from build123d import *
from OCP.BRepAlgoAPI import BRepAlgoAPI_Cut
from OCP.TopTools import TopTools_ListOfShape

# Parameters (mm, degrees)
SKETCH1_R               = 10
BOSS_EXTRUDE2_DEPTH     = 30
SKETCH4_R               = 10
CUT_EXTRUDE1_DEPTH      = 15
CHAMFER1_SIZE           = 20
CUT_EXTRUDE2_DEPTH      = 174.638139858
CUT_EXTRUDE2_DEPTH_BACK = 174.638139858
BOSS_EXTRUDE3_DEPTH     = 45
CUT_EXTRUDE3_DEPTH      = 198.547978004
CUT_EXTRUDE3_DEPTH_BACK = 15
SKETCH6_3_R             = 9
SKETCH8_W               = 15
SKETCH8_H               = 36
BOSS_EXTRUDE4_DEPTH     = 45.000002
SKETCH10_R              = 9
CUT_EXTRUDE4_DEPTH      = 198.547978004
BOSS_EXTRUDE5_DEPTH     = 10
CHAMFER2_SIZE           = 12
CUT_EXTRUDE5_DEPTH      = 40
CUT_EXTRUDE6_DEPTH      = 217.852953896
CUT_EXTRUDE6_DEPTH_BACK = 217.852953896
SKETCH14_W              = 100
SKETCH14_H              = 60
CUT_EXTRUDE7_DEPTH      = 145.655593904
CUT_EXTRUDE7_DEPTH_BACK = 10
SKETCH16_R              = 10
CUT_EXTRUDE8_DEPTH      = 15


# Some blends are built 0.0001 mm under size
with BuildPart() as part:
    # Sketch1 → Boss-Extrude2 (new, symmetric)
    # profile 1 of 3: a face of its own
    with BuildSketch(Plane.XY):
        Polygon((25, -10), (-4.997737685, -45.002262315), (-25, -25), (-25, 25), (25, 25), align=None)
        Circle(SKETCH1_R, mode=Mode.SUBTRACT)
    # profile 2 of 3: a face of its own
    with BuildSketch(Plane.XY):
        Polygon((45, -10), (25, -10), (-4.997737685, -45.002262315), (45.002262315, -45.002262315), (75, -41.079226753), (75, -2.548159698), align=None)
    # profile 3 of 3: a face of its own
    with BuildSketch(Plane.XY):
        Polygon((130, 11.113547523), (75, -2.548159698), (75, -41.079226753), (130, -33.886452477), (165, -33.886452477), (165, 11.113547523), align=None)
    extrude(amount=BOSS_EXTRUDE2_DEPTH, both=True)

    # Sketch4 → Cut-Extrude1 (cut, symmetric)
    with BuildSketch(Plane.XY):
        Polygon((25, -10), (-4.997737685, -45.002262315), (-25, -25), (-25, 25), (25, 25), align=None)
        Circle(SKETCH4_R, mode=Mode.SUBTRACT)
    extrude(amount=CUT_EXTRUDE1_DEPTH, both=True, mode=Mode.SUBTRACT)

    # Chamfer1
    chamfer1_edges = [part.edges().sort_by_distance(p)[0] for p in [
        (25, -10, -22.5),
        (25, -10, 22.5),
    ]]
    chamfer(chamfer1_edges, length=CHAMFER1_SIZE - 0.0001)  # a hair under: the kernel refuses the full size

    # Sketch5 → Cut-Extrude2 (cut, two sides: drawn at the far end of the back side and taken through both)
    with BuildSketch(Plane(origin=(0, 0, 0), x_dir=(1, 0, 0), z_dir=(0, 1, 0)).offset(-CUT_EXTRUDE2_DEPTH_BACK)):
        Polygon((165, -30), (165, -18), (55.074227224, -30), align=None)
        Polygon((165, 18), (165, 30), (55.074227224, 30), align=None)
    extrude(amount=CUT_EXTRUDE2_DEPTH + CUT_EXTRUDE2_DEPTH_BACK, mode=Mode.SUBTRACT)

    # Sketch6 → Boss-Extrude3 (add)
    with BuildSketch(Plane(origin=(165, 0, 0), x_dir=(0, 0, -1), z_dir=(1, 0, 0))):
        with BuildLine():
            Line((-18, -33.886452477), (18, -33.886452477))
            Line((18, -33.886452477), (18, -17.886452477))
            ThreePointArc((18, -17.886452477), (0, -25.375680921), (-18, -17.886452477))
            Line((-18, -17.886452477), (-18, -33.886452477))
        make_face()
    extrude(amount=BOSS_EXTRUDE3_DEPTH)

    # Sketch6<3> → Cut-Extrude3 (cut, two sides: drawn at the far end of the back side and taken through both)
    with BuildSketch(Plane(origin=(165, 0, 0), x_dir=(0, 0, -1), z_dir=(1, 0, 0)).offset(-CUT_EXTRUDE3_DEPTH_BACK)):
        with Locations(Location((0, -1.886452477, 0), (0, 0, 90))):
            Circle(SKETCH6_3_R)
    extrude(amount=CUT_EXTRUDE3_DEPTH + CUT_EXTRUDE3_DEPTH_BACK, mode=Mode.SUBTRACT)

    # Sketch8 → Boss-Extrude4 (add)
    with BuildSketch(Plane.XZ.offset(33.886452477)):
        with Locations((202.5, 0)):
            Rectangle(SKETCH8_W, SKETCH8_H)
    extrude(amount=-BOSS_EXTRUDE4_DEPTH)

    # Sketch10 → Cut-Extrude4 (cut, through all)
    with BuildSketch(Plane(origin=(165, 0, 0), x_dir=(0, 0, -1), z_dir=(1, 0, 0))):
        with Locations(Location((0, -1.886452477, 0), (0, 0, 90))):
            Circle(SKETCH10_R)
    extrude(amount=CUT_EXTRUDE4_DEPTH, mode=Mode.SUBTRACT)

    # Sketch11 → Boss-Extrude5 (add)
    with BuildSketch(Plane.XZ.offset(33.886452477)):
        Polygon((130, 21.82076004), (130, -21.82076004), (165, -18), (210, -18), (210, 18), (165, 18), align=None)
    extrude(amount=BOSS_EXTRUDE5_DEPTH)

    # Chamfer2
    # the kernel refuses this chamfer: 12 mm, written as the material it takes off along each edge
    with BuildSketch(Plane(origin=(130, -43.886452477, 52.680955896), x_dir=(0, 1, 0), z_dir=(0, 0, -1))) as chamfer2_piece_1_section:
        Polygon((CHAMFER2_SIZE, 0), (0, CHAMFER2_SIZE), (0, 0), align=None)
    chamfer2_piece_1 = extrude(amount=105.361911791, mode=Mode.PRIVATE)
    chamfer2_piece_1 = split(chamfer2_piece_1, bisect_by=Plane(origin=(128.714213423, -34.054604706, 52.680955896), z_dir=(0.1296735244167249, -0.9915567442488328, 0)), keep=Keep.TOP, mode=Mode.PRIVATE)
    add(chamfer2_piece_1, mode=Mode.SUBTRACT)

    # Sketch13 → Cut-Extrude5 (cut)
    with BuildSketch(Plane.XY.offset(18)):
        with BuildLine():
            Line((165, -17.886452477), (195, -17.886452477))
            ThreePointArc((195, -17.886452477), (180, -25.224548687), (165, -17.886452477))
        make_face()
    extrude(amount=-CUT_EXTRUDE5_DEPTH, mode=Mode.SUBTRACT)

    # Sketch14 → Cut-Extrude6 (cut, two sides: drawn at the far end of the back side and taken through both)
    with BuildSketch(Plane(origin=(0, 0, 0), x_dir=(1, 0, 0), z_dir=(0, 1, 0)).offset(-CUT_EXTRUDE6_DEPTH_BACK)):
        with Locations((25, 0)):
            Rectangle(SKETCH14_W, SKETCH14_H)
    extrude(amount=CUT_EXTRUDE6_DEPTH + CUT_EXTRUDE6_DEPTH_BACK, mode=Mode.SUBTRACT)

    # Sketch16 → Cut-Extrude7 (cut, two sides: drawn at the far end of the back side and taken through both)
    with BuildSketch(Plane.ZY.offset(-75).offset(-CUT_EXTRUDE7_DEPTH_BACK)):
        with Locations(Location((0, -20.03233432, 0), (0, 0, 180))):
            Circle(SKETCH16_R)
    extrude(amount=CUT_EXTRUDE7_DEPTH + CUT_EXTRUDE7_DEPTH_BACK, mode=Mode.SUBTRACT)


with BuildPart() as cut_extrude8_tool:
    # Sketch17 → Cut-Extrude8 (new body)
    with BuildSketch(Plane(origin=(210, 0, 0), x_dir=(0, 0, -1), z_dir=(1, 0, 0))):
        with BuildLine():
            Line((-6.182771984, 11.113547523), (-3.573497387, 6.373699848))
            ThreePointArc((-3.573497387, 6.373699848), (-0.036026842, 7.113475415), (3.507252904, 6.402044194))
            Line((3.507252904, 6.402044194), (6.304774933, 11.113547523))
            Line((6.304774933, 11.113547523), (-6.182771984, 11.113547523))
        make_face()
    extrude(amount=-CUT_EXTRUDE8_DEPTH)


with BuildPart() as part_1:
    add(part.part)

    # Cut-Extrude8: cut by cut_extrude8_tool, with a tolerance
    cut_extrude8_stock = TopTools_ListOfShape()
    cut_extrude8_stock.Append(part_1.part.wrapped)
    cut_extrude8_tools = TopTools_ListOfShape()
    cut_extrude8_tools.Append(cut_extrude8_tool.part.wrapped)
    cut_extrude8_cut = BRepAlgoAPI_Cut()
    cut_extrude8_cut.SetArguments(cut_extrude8_stock)
    cut_extrude8_cut.SetTools(cut_extrude8_tools)
    cut_extrude8_cut.SetFuzzyValue(0.00001)
    cut_extrude8_cut.Build()
    add(Compound.cast(cut_extrude8_cut.Shape()).solids(), mode=Mode.REPLACE)


solid = part_1.part
Model file for the job. Use its own axes, mm. A direction names the side the tool comes from. Give positions to 0.01 mm unless a question says otherwise; leave off trailing zeros. Write each loop counter-clockwise with the first axis right and the second up, starting at its lowest first coordinate (ties: lowest second). Pieces come first, ordered by that corner, then holes. Notation, with made-up numbers: M -16.75,58 L 7.25,58 A34 ccw 7.25,91 Z; hole C 18,-19 d8. An arc over 180 degrees is marked long. One line per item, written item: value. Start each with the question number.
Q1. Saw through at B-B, the plane z = 0. Write the cut outline in (x, y), plus the area to 3 significant figures.
Q2. Drop flat-ended pins along their axis: pin 1 Ø16 at (y, z) = (-1.89, 0) entering from -X; pin 2 Ø8 at (x, y) = (112.5, -4) entering from -Z; pin 3 Ø5.5 at (y, z) = (-4, 1.5) entering from +X; pin 4 Ø10 at (y, z) = (-22.5, 2) entering from -X. Give the stop position or say it passes through.
Q3. Probe probe 1 along X at (y, z) = (-17.5, -13.5); probe 2 along Y at (x, z) = (160, 0); probe 3 along X at (y, z) = (-13, -4). List the from-to ranges inside material, lowest first. Write a range as [from, to].
Q4. Saw through at C-C, the plane y = -5.5. Write the cut outline in (x, z), plus the area to 3 significant figures.
Q5. Saw through at D-D, the plane x = 191. Write the cut outline in (y, z).
Q6. Saw through at A-A, the plane y = -14. Write the cut outline in (x, z).
Q7. Two-plate mould, pull along X, no slides. Class faces 1 (the cylindrical face through (80.07, -29.947, 1.302)), 2 (the cylindrical face through (179.79, -25.374, -0.28)), 3 (the flat face through (136.813, -38.699, 0.303)), 4 (the flat face through (150, -2, 0)): +X half, -X half, draft (parallel to the pull), parting line (faces both ways), or undercut.
Q8. 3-axis set-ups, long thin cutter, end or side, ignore diameter. For faces 5 (the flat face through (85, -20, 0)), 6 (the flat face through (202.605, 8.725, -4.886)), 7 (the flat face through (192, -22, -18)), 8 (the flat face through (193, -22, 18)): which of +Z, -Z, +X, -X, +Y, -Y reach the whole face in a straight line?
Output values:
1. outline: M 75,-41.08 L 131.77,-33.66 L 142,-43.89 L 210,-43.89 L 210,-10.89 L 195,-10.89 L 195,-25.38 L 165,-25.38 L 165,-10.89 L 150,-10.89 L 150,7.11 L 165,7.11 L 165,11.11 L 130,11.11 L 75,-2.55 L 75,-10.03 L 85,-10.03 L 85,-30.03 L 75,-30.03 Z
1. area: 4,730 mm²
2. pin 1: stops at x = 75
2. pin 2: stops at z = -24.17
2. pin 3: stops at x = 150
2. pin 4: stops at x = 85
3. probe 1: x = [75, 165], [195, 210]
3. probe 2: y = [-43.89, -10.89], [7.11, 11.11]
3. probe 3: x = [85, 165], [195, 210]
4. outline: M 75,-27.82 L 165,-18 L 165,-8.24 L 150,-8.24 L 150,8.24 L 165,8.24 L 165,18 L 75,27.82 Z; M 195,-18 L 210,-18 L 210,-8.24 L 195,-8.24 Z; M 195,8.24 L 210,8.24 L 210,18 L 195,18 Z
4. area: 4,170 mm²
5. outline: M -43.89,-18 L -21.72,-18 L -21.72,-13.13 A25.38 cw -21.72,13.13 L -21.72,18 L -43.89,18 Z
6. outline: M 75,-27.82 L 165,-18 L 165,18 L 75,27.82 L 75,7.98 L 85,7.98 L 85,-7.98 L 75,-7.98 Z; M 195,-18 L 210,-18 L 210,18 L 195,18 Z
7. face 1: draft
7. face 2: undercut
7. face 3: undercut
7. face 4: +X half
8. face 5: -X
8. face 6: +X, +Y
8. face 7: -Z, +X, +Y, -Y
8. face 8: +Z, +X, +Y, -Y
